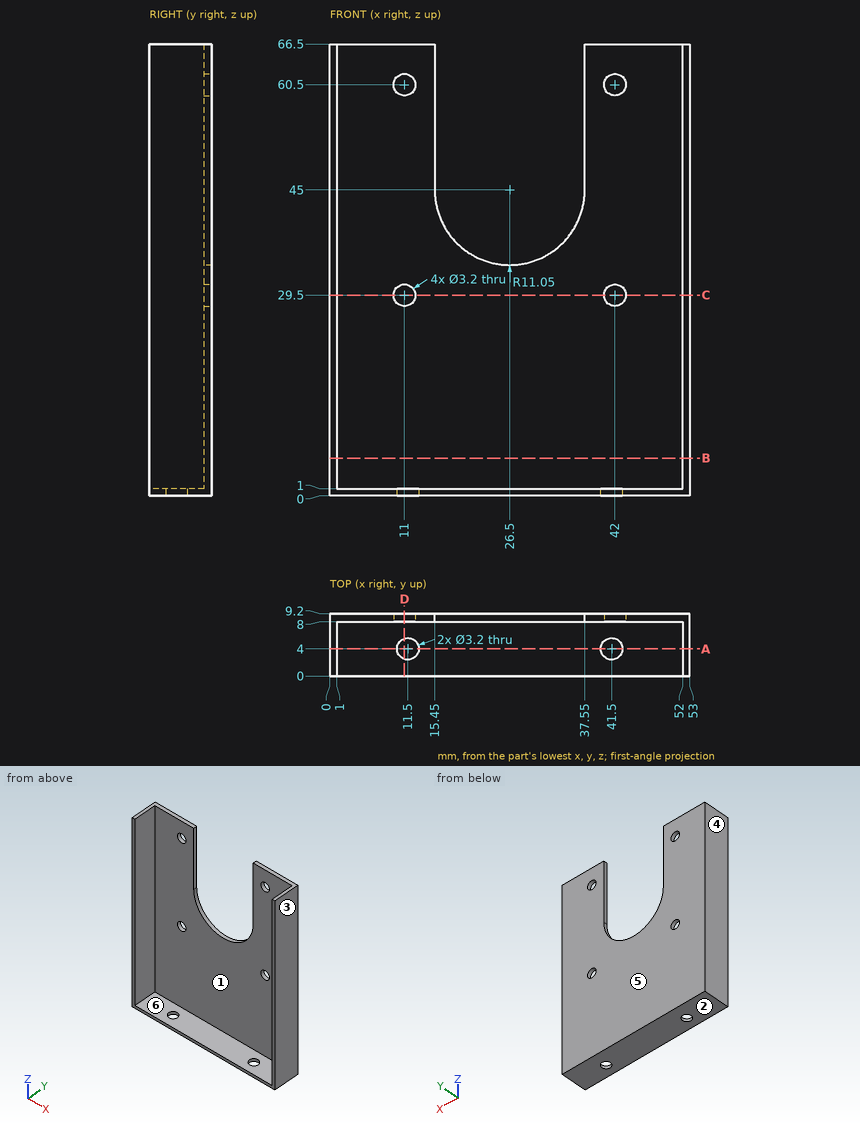
For this review, use the dimensioned drawing (mm, ordinates from the lowest corner) and the shaded views. A direction names the side the tool comes from. Round coordinates to 2 decimals unless told otherwise and drop trailing zeros. Loops run counter-clockwise (first coordinate to the right, second up) from the corner with the lowest first, then second, coordinate; pieces in that order, holes last. Notation, with made-up numbers: M 89,-21 L 94,-21 A13 ccw 94,-12 Z; hole C 19.5,27 d9. An arc over 180 degrees is marked long. Answer as CSV lines item,"result".
1. We need section D-D (x = 11). Give the boundary of the cut face in (y, z).
Outcome:
outline,"M 0,0 L 2.48,0 L 2.48,1 L 0,1 Z; M 5.52,0 L 9.2,0 L 9.2,27.9 L 8,27.9 L 8,1 L 5.52,1 Z; M 8,31.1 L 9.2,31.1 L 9.2,58.9 L 8,58.9 Z; M 8,62.1 L 9.2,62.1 L 9.2,66.5 L 8,66.5 Z"
2. We need section B-B (z = 5.5). Give the boundary of the cut face in (x, y), plus the area to 3 significant figures.
Outcome:
outline,"M 0,0 L 1,0 L 1,8 L 52,8 L 52,0 L 53,0 L 53,9.2 L 0,9.2 Z"
area,"79.6 mm2"
3. Insertion check: pin 1 Ø1 at (y, z) = (8.5, 53) entering from -X; pin 2 Ø4 at (x, y) = (11.5, 4) entering from +Z; pin 3 Ø5 at (x, z) = (42, 60.5) entering from -Y; pin 4 Ø3 at (x, z) = (42, 29.5) entering from +Y. Each pin has a flat end and moves straight along its axis. Give the tip position at first contact, or say it passes through.
Outcome:
pin 1,"stops at x = 0"
pin 2,"stops at z = 1"
pin 3,"stops at y = 8"
pin 4,"passes through"
4. Draft analysis for pull direction X (two halves, no side actions). For the marked faces 1, 2, 3 and 4, state which applies: pulls with the +X half, pulls with the -X half, needs draft (parallel to the pull), parting line crosses it, or undercut.
Outcome:
face 1,"undercut"
face 2,"needs draft"
face 3,"pulls with the +X half"
face 4,"pulls with the -X half"
5. For the marked faces 5 and 6, list the 3-axis set-ups (+Z, -Z, +X, -X, +Y, -Y) from which the entire face can be reached by the end or side of a thin tool; tool diameter is ignored.
Outcome:
face 5,"+Z, -Z, +X, -X, +Y"
face 6,"+Z, -Y"
6. To check wall thickness, follow L1, parallel to X at y = 8.8, z = 60.5; L2, parallel to X at y = 8.6, z = 29.5; L3, parallel to X at y = 3, z = 52. State the ranges of each line that lie inside material, in increasing order. Write a range as [from, to].
Outcome:
L1,"x = [0, 9.4], [12.6, 15.45], [37.55, 40.4], [43.6, 53]"
L2,"x = [0, 9.4], [12.6, 40.4], [43.6, 53]"
L3,"x = [0, 1], [52, 53]"
7. We need section A-A (y = 4). Give the boundary of the cut face in (x, z), plus the area to 3 significant figures.
Outcome:
outline,"M 0,0 L 9.9,0 L 9.9,1 L 1,1 L 1,66.5 L 0,66.5 Z; M 13.1,0 L 39.9,0 L 39.9,1 L 13.1,1 Z; M 43.1,0 L 53,0 L 53,66.5 L 52,66.5 L 52,1 L 43.1,1 Z"
area,"178 mm2"
8. We need section C-C (z = 29.5). Give the boundary of the cut face in (x, y).
Outcome:
outline,"M 0,0 L 1,0 L 1,8 L 9.4,8 L 9.4,9.2 L 0,9.2 Z; M 12.6,8 L 40.4,8 L 40.4,9.2 L 12.6,9.2 Z; M 43.6,8 L 52,8 L 52,0 L 53,0 L 53,9.2 L 43.6,9.2 Z"
